```python
from build123d import *

# Parameters (mm, degrees)
F1_DEPTH = 3.175


with BuildPart() as f1:
    # F0 (on Front) → F1 (new body)
    with BuildSketch(Plane.XZ):
        with BuildLine():
            Line((57.15, 0), (63.5, 0))
            ThreePointArc((63.5, 0), (62.82811, 9.21296), (60.826657, 18.230956))
            Line((60.826657, 18.230956), (56.284487, 16.799141))
            Line((56.284487, 16.799141), (55.406307, 19.585005))
            Line((55.406307, 19.585005), (59.923863, 21.009061))
            ThreePointArc((59.923863, 21.009061), (51.370959, 37.326593), (38.493912, 50.502165))
            Line((38.493912, 50.502165), (35.660819, 46.673982))
            Line((35.660819, 46.673982), (33.312867, 48.411612))
            Line((33.312867, 48.411612), (36.130607, 52.219051))
            ThreePointArc((36.130607, 52.219051), (19.619958, 60.392941), (1.457801, 63.483264))
            Line((1.457801, 63.483264), (1.415931, 58.720948))
            Line((1.415931, 58.720948), (-1.504956, 58.746629))
            Line((-1.504956, 58.746629), (-1.463313, 63.483137))
            ThreePointArc((-1.463313, 63.483137), (-19.625201, 60.391237), (-36.13514, 52.215914))
            Line((-36.13514, 52.215914), (-33.369795, 48.338508))
            Line((-33.369795, 48.338508), (-35.747937, 46.64243))
            Line((-35.747937, 46.64243), (-38.498297, 50.498823))
            ThreePointArc((-38.498297, 50.498823), (-51.374199, 37.322134), (-59.925687, 21.003859))
            Line((-59.925687, 21.003859), (-55.409394, 19.492401))
            Line((-55.409394, 19.492401), (-56.336421, 16.722408))
            Line((-56.336421, 16.722408), (-60.82824, 18.225675))
            ThreePointArc((-60.82824, 18.225675), (-62.82851, 9.210233), (-63.5, 0))
            Line((-63.5, 0), (-57.15, 0))
            Line((-57.15, 0), (-57.15, 2.9718))
            Line((-57.15, 2.9718), (-53.893126, 2.9718))
            ThreePointArc((-53.893126, 2.9718), (0, 53.975), (53.893126, 2.9718))
            Line((53.893126, 2.9718), (53.975, 2.9718))
            Line((53.975, 2.9718), (57.15, 2.9718))
            Line((57.15, 2.9718), (57.15, 0))
        make_face()
    extrude(amount=F1_DEPTH)


solid = f1.part
```
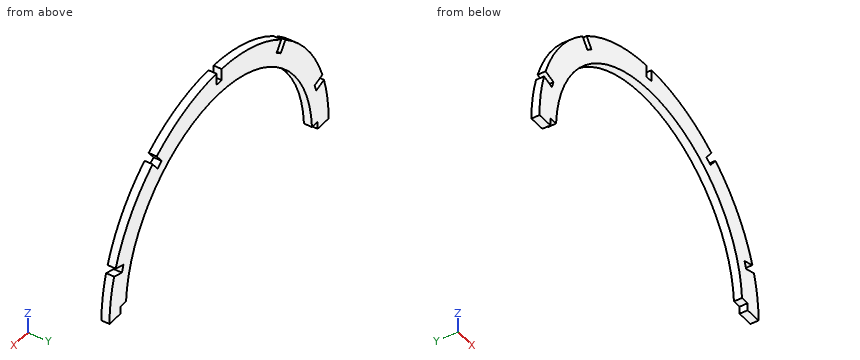
Source: CAD feature listing. Evaluate the final solid. Frame: model axes, mm. Give positions to 0.01 mm unless a question says otherwise; leave off trailing zeros. Write each loop counter-clockwise with the first axis right and the second up, starting at its lowest first coordinate (ties: lowest second). Pieces come first, ordered by that corner, then holes.
1. First-contact query: pin 1 (1.5 mm diameter, centred on y = -2, z = 41.5, fed in from +X); pin 2 (1 mm diameter, centred on x = 23.5, y = -1, fed in from +Z); pin 3 (1.6 mm diameter, centred on x = -56, y = -1, fed in from -Z). Flat tips, straight axial feed; report the tip coordinate or a pass-through.
2. Material intervals for line 1 along X through (y, z) = (-2.1, 47.5); line 2 along Z through (x, y) = (35, -1.9); line 3 along Z through (x, y) = (-57, -1), sorted ascending.
3. Section query A-A (z = 40.5). Return the cut outline in (x, y) (3 decimals), then the cut area to 3 significant figures.
4. Section query C-C (z = 34). Return the cut outline in (x, y) (3 decimals).
5. Section query D-D (x = 0). Return the cut outline in (y, z) (3 decimals).
Output values:
1. pin 1: stops at x = 48.7
1. pin 2: stops at z = 59.19
1. pin 3: stops at z = 2.97
2. line 1: x = -42.14 to -36.36, -34.55 to -25.63, 25.63 to 34.54, 36.27 to 42.14
2. line 2: z = 41.09 to 47.16, 50.69 to 52.98
2. line 3: z = 2.97 to 16.94, 20.02 to 27.99
3. outline: (-48.908, -3.175) - (-35.68, -3.175) - (-35.68, 0) - (-48.908, 0) - close; (35.68, -3.175) - (48.908, -3.175) - (48.908, 0) - (35.68, 0) - close
3. area: 84.0 mm2
4. outline: (-53.631, -3.175) - (-41.92, -3.175) - (-41.92, 0) - (-53.631, 0) - close; (41.92, -3.175) - (53.631, -3.175) - (53.631, 0) - (41.92, 0) - close
5. outline: (-3.175, 53.975) - (0, 53.975) - (0, 58.733) - (-3.175, 58.733) - close
